Model file for the job. Use its own axes, mm. Round coordinates to 2 decimals unless told otherwise and drop trailing zeros. Loops run counter-clockwise (first coordinate to the right, second up) from the corner with the lowest first, then second, coordinate; pieces in that order, holes last. Notation, with made-up numbers: M -19,-11 L 21,-11 A22 cw 21,-5 Z; hole C 75,76 d4. An arc over 180 degrees is marked long. Use a Markdown table: item, result. Add a question column.
Item 1: Saw through at D-D on y = 5. Write the cut outline in (x, z).
Item 2: Saw through at A-A on x = 5. Write the cut outline in (y, z).
Item 3: Two-plate mould, pull along Y, no slides. Class faces 1 (the flat face through (5, 0, 5)), 2 (the cylindrical face through (4.792, 16.586, 5.07)), 3 (the flat face through (5, 20, 5)), 4 (the flat face through (0, 10, 5)): +Y half, -Y half, draft (parallel to the pull), parting line (faces both ways), or undercut.
Item 4: Saw through at B-B on z = 5. Write the cut outline in (x, y), then the cut area to 3 significant figures.
Item 5: Wall check: L1, parallel to Z at x = 5.5, y = 5; L2, parallel to Y at x = 5, z = 7.25; L3, parallel to Y at x = 4.5, z = 2.75. Give the ranges that are in metal, low to high. Write a range as from..to.
Item 6: Saw through at C-C on y = 15. Write the cut outline in (x, z).
```python
from build123d import *

# Parameters (mm, degrees)
SKETCH_1_W          = 10
SKETCH_1_H          = 20
EXTRUDE_1_DEPTH     = 10
SKETCH_2_R          = 2.6
CUT_EXTRUDE_1_DEPTH = 25.494897428
SKETCH_3_R          = 1.6
CUT_EXTRUDE_2_DEPTH = 10


with BuildPart() as part:
    # ｽｹｯﾁ1 → ﾎﾞｽ - 押し出し1 (new body)
    with BuildSketch(Plane.XY):
        with Locations((5, 10)):
            Rectangle(SKETCH_1_W, SKETCH_1_H)
    extrude(amount=EXTRUDE_1_DEPTH)

    # ｽｹｯﾁ2 → ｶｯﾄ - 押し出し1 (cut, through all)
    with BuildSketch(Plane(origin=(10, 0, 0), x_dir=(0, 0, -1), z_dir=(1, 0, 0))):
        with Locations(Location((-5, 5, 0), (0, 0, 90))):
            Circle(SKETCH_2_R)
    extrude(amount=-CUT_EXTRUDE_1_DEPTH, mode=Mode.SUBTRACT)

    # ｽｹｯﾁ3 → ｶｯﾄ - 押し出し2 (cut)
    with BuildSketch(Plane.XY.offset(10)):
        with Locations((5, 15)):
            Circle(SKETCH_3_R)
    extrude(amount=-CUT_EXTRUDE_2_DEPTH, mode=Mode.SUBTRACT)


solid = part.part
```
Entries:
| question | item | result |
|---|---|---|
| 1 | outline | M 0,0 L 10,0 L 10,2.4 L 0,2.4 Z; M 0,7.6 L 10,7.6 L 10,10 L 0,10 Z |
| 2 | outline | M 0,0 L 13.4,0 L 13.4,10 L 0,10 Z; M 16.6,0 L 20,0 L 20,10 L 16.6,10 Z; hole C 5,5 d5.2 |
| 3 | face 1 | -Y half |
| 3 | face 2 | undercut |
| 3 | face 3 | +Y half |
| 3 | face 4 | draft |
| 4 | outline | M 0,0 L 10,0 L 10,2.4 L 0,2.4 Z; M 0,7.6 L 10,7.6 L 10,20 L 0,20 Z; hole C 5,15 d3.2 |
| 4 | area | 140 mm2 |
| 5 | L1 | 0..2.4, 7.6..10 |
| 5 | L2 | 0..3.7, 6.3..13.4, 16.6..20 |
| 5 | L3 | 0..3.7, 6.3..13.48, 16.52..20 |
| 6 | outline | M 0,0 L 3.4,0 L 3.4,10 L 0,10 Z; M 6.6,0 L 10,0 L 10,10 L 6.6,10 Z |
